Geometry: final body of the model. Coordinates: model frame, mm. Round coordinates to 2 decimals unless told otherwise and drop trailing zeros. Loops run counter-clockwise (first coordinate to the right, second up) from the corner with the lowest first, then second, coordinate; pieces in that order, holes last. Notation, with made-up numbers: (4, 2) - (32, 2) arc R36 ccw to (32, 36) - close; hole circle Ø10 at (-32.5, -35.5). An arc over 180 degrees is marked (long way). Answer in a Markdown table with one row per item. Add a question column.
from build123d import *

# Parameters (mm, degrees)
F0_W     = 25.4
F0_H     = 254
F1_DEPTH = 6.35
F3_D     = 4.4958
F5_D     = 4.4958


with BuildPart() as f1:
    # F0 (on Right) → F1 (new body)
    with BuildSketch(Plane.YZ):
        with Locations((12.7, 127)):
            Rectangle(F0_W, F0_H)
    extrude(amount=-F1_DEPTH)

    # F3 (through all)
    with Locations(Plane.YZ):
        with Locations((8.46666582, 247.65), (16.93333418, 247.65)):
            Hole(F3_D / 2)

    # F5 (through all)
    with Locations(Plane.YZ):
        with Locations((12.7, 43.391666328), (12.7, 21.695833164)):
            Hole(F5_D / 2)


solid = f1.part
1) Material intervals for line 1 along Z through (x, y) = (-6, 12.25); line 2 along Y through (x, z) = (-4, 247.65); line 3 along Z through (x, y) = (-2, 12.7), sorted ascending. Write a range as from..to.
2) Section A-A, the plane z = 247.65. Return the cut outline in (x, y), and give its area (3 significant figures).
3) Pull-direction query (Z, two-part tool) for faces 1 (the cylindrical face through (-3.22, 13.19, 19.5)), 2 (the flat face through (-6.35, 13, 129)), 3 (the flat face through (-3, 13, 0)); classes: pulls with the +Z half, pulls with the -Z half, needs draft (parallel to the pull), parting line crosses it, or undercut.
Evaluation:
| question | item | result |
|---|---|---|
| 1 | line 1 | z = 0..19.49, 23.9..41.19, 45.59..254 |
| 1 | line 2 | y = 0..6.22, 10.71..14.69, 19.18..25.4 |
| 1 | line 3 | z = 0..19.45, 23.94..41.14, 45.64..254 |
| 2 | outline | (-6.35, 0) - (0, 0) - (0, 6.22) - (-6.35, 6.22) - close; (-6.35, 10.71) - (0, 10.71) - (0, 14.69) - (-6.35, 14.69) - close; (-6.35, 19.18) - (0, 19.18) - (0, 25.4) - (-6.35, 25.4) - close |
| 2 | area | 104 mm² |
| 3 | face 1 | undercut |
| 3 | face 2 | needs draft |
| 3 | face 3 | pulls with the -Z half |
